Check sheet for the modelled part. Datum: model origin and axes. Units: mm. A direction names the side the tool comes from. Give positions to 0.01 mm unless a question says otherwise; leave off trailing zeros. Order: outer loops, then holes, each group sorted by start corner. A loop starts at its lowest first (then second) coordinate and runs counter-clockwise, first axis right, second up. Notation, with made-up numbers: (-26.75, 0) -> (-20.75, 0) arc R15 ccw to (-20.75, 17) -> close; hole circle Ø10 at (25.25, 66). An arc over 180 degrees is marked (long way). Write each question's results on one line, items separated by ' | '.
from build123d import *

# Parameters (mm, degrees)
PAD_DEPTH    = 10.19
SKETCH002_R  = 6
PAD001_DEPTH = 28.5


with BuildPart() as part:
    # Sketch → Pad (new body)
    with BuildSketch(Plane.XY):
        Polygon((0, 10.39), (-8.998004, 5.195), (-8.998004, -5.195), (0, -10.39), (8.998004, -5.195), (8.998004, 5.195), align=None)
    extrude(amount=PAD_DEPTH)

    # Sketch002 (on DatumPlane) → Pad001 (join)
    with BuildSketch(Plane(origin=(0, 0, 0), x_dir=(-1, 0, 0), z_dir=(0, 0, -1))):
        Circle(SKETCH002_R)
    extrude(amount=PAD001_DEPTH)

    # Sketch001 → Groove (revolve, cut)
    with BuildSketch(Plane.YZ):
        Polygon((-8.998004, 10.19), (-19.388004, 10.19), (-19.388004, 4.191331), align=None)
        Polygon((-8.998004, 0), (-19.388004, 0), (-19.388004, 5.998669), align=None)
    revolve(axis=Axis((0, 0, 0), (0, 0, 1)), mode=Mode.SUBTRACT)


solid = part.part
1. Access from +Z, -Z, +X, -X, +Y, -Y to the whole of each face (thin tool, end or side, straight path). Record for faces 1 (the flat face through (2, -6, 0)), 2 (the flat face through (-4.562, -7.756, 5.024)).
Verdict:
face 1: -Z | face 2: +Z, -Z, -X, -Y
2. Material ranges on probe 1 along Z at (x, y) = (7.75, -2); probe 2 along Y at (x, z) = (-3, -20); probe 3 along Y at (x, z) = (4, -17), recorded low to high. Write a range as from..to.
Verdict:
probe 1: z = 0..10.19 | probe 2: y = -5.2..5.2 | probe 3: y = -4.47..4.47
3. Section check A-A on z = -5. Record the cut outline in (x, y).
Verdict:
outline: circle Ø12 at (0, 0)
4. Gauge pin test, flat ends, axial feed: pin 1 Ø3 at (y, z) = (-5, -23) entering from -X; pin 2 Ø1 at (x, z) = (-5, -15) entering from -Y; pin 3 Ø1.5 at (y, z) = (-1, -3) entering from -X. Record the tip position at first contact, or that the pin passes through.
Verdict:
pin 1: stops at x = -4.87 | pin 2: stops at y = -3.97 | pin 3: stops at x = -5.99
